Geometry: see drawing. Coordinates: mm, zero at the bounding-box minimum. Coordinates: 2 decimals unless noted, no trailing zeros. Loops run counter-clockwise (first coordinate to the right, second up) from the corner with the lowest first, then second, coordinate; pieces in that order, holes last. Notation, with made-up numbers: (-39, -11) - (18, -11) arc R12 ccw to (18, 4) - close; hole circle Ø3 at (12.5, 8.5). An arc over 180 degrees is marked (long way). Answer in a Markdown table with one row per item.
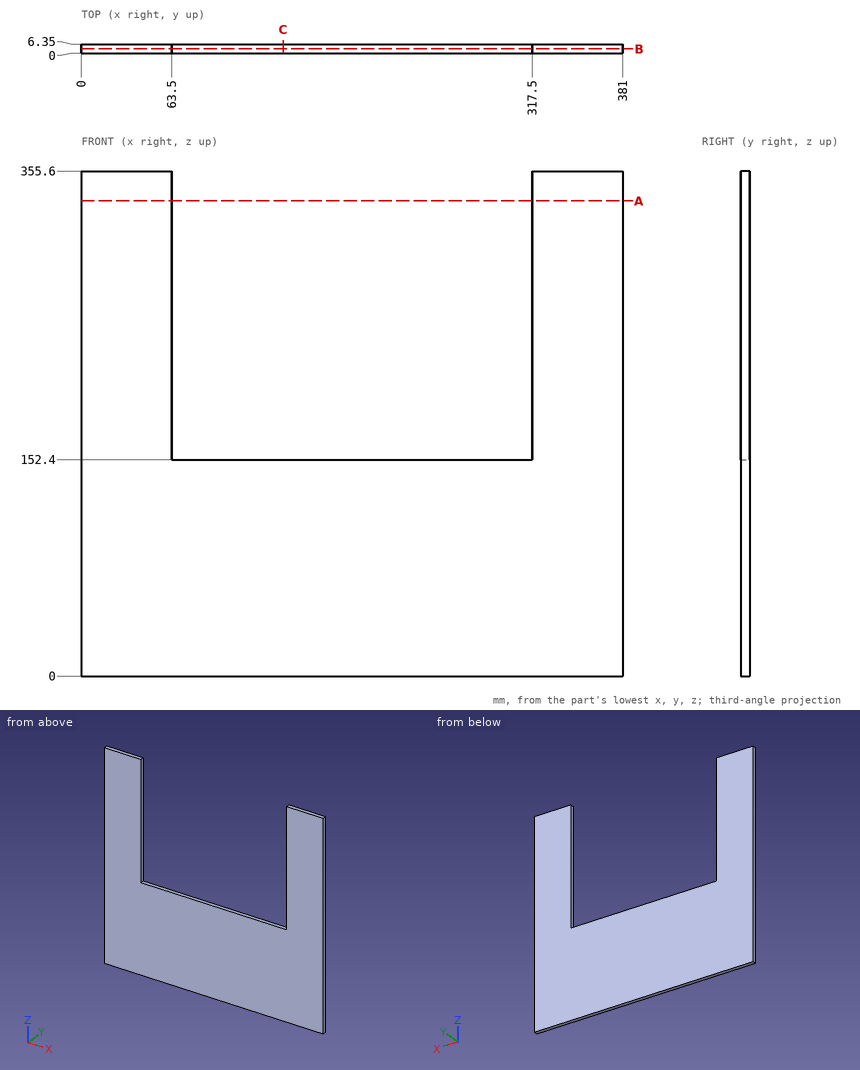
(1) Cut plane C-C on x = 142. Output: boundary loops of the cut face in (y, z).
Verdict:
| item | result |
|---|---|
| outline | (0, 0) - (6.35, 0) - (6.35, 152.4) - (0, 152.4) - close |
(2) Cut plane A-A on z = 334.5. Output: boundary loops of the cut face in (x, y), then the cut area to 3 significant figures.
Verdict:
| item | result |
|---|---|
| outline | (0, 0) - (63.5, 0) - (63.5, 6.35) - (0, 6.35) - close; (317.5, 0) - (381, 0) - (381, 6.35) - (317.5, 6.35) - close |
| area | 806 mm² |
(3) First-contact query: pin 1 Ø1.5 at (x, y) = (108.5, 3) entering from +Z. Flat tip, straight axial feed; report the tip coordinate or a pass-through.
Verdict:
| item | result |
|---|---|
| pin 1 | stops at z = 152.4 |
(4) Cut plane B-B on y = 3. Output: boundary loops of the cut face in (x, z).
Verdict:
| item | result |
|---|---|
| outline | (0, 0) - (381, 0) - (381, 355.6) - (317.5, 355.6) - (317.5, 152.4) - (63.5, 152.4) - (63.5, 355.6) - (0, 355.6) - close |
(5) Ray query, probe 1 along X at (y, z) = (4.5, 294.5); probe 2 along Z at (x, y) = (67.5, 2.5). Return the intervals inside material, ascending.
Verdict:
| item | result |
|---|---|
| probe 1 | x = 0 to 63.5, 317.5 to 381 |
| probe 2 | z = 0 to 152.4 |
